Design review of the part built by this model. Coordinates are the model's own, in mm. Face numbers are marked on the shaded views. A direction names the side the tool comes from. Round coordinates to 2 decimals unless told otherwise and drop trailing zeros. Loops run counter-clockwise (first coordinate to the right, second up) from the corner with the lowest first, then second, coordinate; pieces in that order, holes last. Notation, with made-up numbers: M 87.5,40.5 L 134.5,40.5 A21 cw 134.5,73.5 Z; hole C 17.25,10.5 d1. An arc over 180 degrees is marked long. Answer as CSV lines item,"result". Start each with the question number.
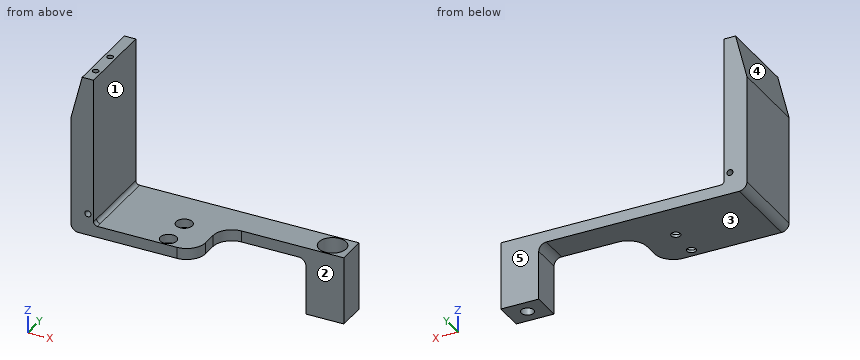
from build123d import *

# Parameters (mm, degrees)
SKETCH_1_W                = 40
SKETCH_1_H                = 10
EXTRUDE_1_DEPTH           = 3
SKETCH_2_W                = 3
SKETCH_2_H                = 10
EXTRUDE_2_DEPTH           = 39.5
EXTRUDE_3_DEPTH           = 10
FILLET_1_R                = 1
SKETCH_4_W                = 40
SKETCH_4_H                = 3
EXTRUDE_4_DEPTH           = 10
HOLE_WIZARD_1_D           = 2.4
HOLE_WIZARD_1_DEPTH       = 3.2
HOLE_WIZARD_1_CBORE_D     = 4.3
HOLE_WIZARD_1_CBORE_DEPTH = 2.3
HOLE_WIZARD_1_TIP         = 0.721032743
HOLE_WIZARD_M2_1_D        = 1.6
HOLE_WIZARD_M2_1_DEPTH    = 5.2
HOLE_WIZARD_M2_1_TIP      = 0.480688495
SKETCH_12_W               = 40
SKETCH_12_H               = 8.5
CUT_EXTRUDE_1_DEPTH       = 43.5
SKETCH_13_W               = 3
SKETCH_13_H               = 21.5
EXTRUDE_5_DEPTH           = 5
SKETCH_14_W               = 3
SKETCH_14_H               = 7.8
EXTRUDE_6_DEPTH           = 27
EXTRUDE_8_DEPTH           = 10
SKETCH_18_W               = 10.684104654
SKETCH_18_H               = 46.640580652
CUT_EXTRUDE_2_DEPTH       = 30
SKETCH_22_W               = 10
SKETCH_22_H               = 7.8
EXTRUDE_9_DEPTH           = 15
SKETCH_23_R               = 3.6
CUT_EXTRUDE_3_DEPTH       = 5
HOLE_WIZARD_M4_1_D        = 3.3
FILLET_2_R                = 2
SKETCH_26_W               = 5
SKETCH_26_H               = 13.7
CUT_EXTRUDE_4_DEPTH       = 8
EXTRUDE_10_DEPTH          = 10
EXTRUDE_11_DEPTH          = 1.5
HOLE_WIZARD_M2_2_D        = 1.6
HOLE_WIZARD_M2_2_DEPTH    = 5.2
HOLE_WIZARD_M2_2_TIP      = 0.480688495
HOLE_WIZARD_M2_3_D        = 1.6
HOLE_WIZARD_M2_3_DEPTH    = 5.2
HOLE_WIZARD_M2_3_TIP      = 0.480688495
HOLE_WIZARD_M2_4_D        = 1.6
HOLE_WIZARD_M2_4_DEPTH    = 5.2
HOLE_WIZARD_M2_4_TIP      = 0.480688495
FILLET_3_R                = 2
FILLET_4_R                = 5


with BuildPart() as part:
    # 草图1 → 凸台-拉伸1 (new body)
    with BuildSketch(Plane.XY):
        Rectangle(SKETCH_1_W, SKETCH_1_H)
    extrude(amount=EXTRUDE_1_DEPTH)

    # 草图2 → 凸台-拉伸2 (add)
    with BuildSketch(Plane.XY.offset(3)):
        with Locations((-8.5, 0)):
            Rectangle(SKETCH_2_W, SKETCH_2_H)
    extrude(amount=EXTRUDE_2_DEPTH)

    # 草图3 → 凸台-拉伸3 (add)
    with BuildSketch(Plane(origin=(0, 5, 0), x_dir=(1, 0, 0), z_dir=(0, 1, 0))):
        Polygon((-20, -3), (-10, -42.5), (-10, -30.276150361), (-16.905354522, -3), align=None)
    extrude(amount=-EXTRUDE_3_DEPTH)

    # 圆角1
    fillet_1_edges = [part.edges().sort_by_distance(p)[0] for p in [
        (-7, 0, 3),
    ]]
    fillet(fillet_1_edges, radius=FILLET_1_R)

    # 草图4 → 凸台-拉伸4 (add)
    with BuildSketch(Plane(origin=(0, 5, 0), x_dir=(1, 0, 0), z_dir=(0, 1, 0))):
        with Locations((0, -1.5)):
            Rectangle(SKETCH_4_W, SKETCH_4_H)
    extrude_4 = extrude(amount=EXTRUDE_4_DEPTH)

    # 镜向1: 凸台-拉伸4 across plane
    add(extrude_4.mirror(Plane.ZX))

    # 打孔尺寸(%根据)内六角圆柱头螺钉的类型1
    with Locations(Plane.XY.offset(3)):
        with Locations((11.5, 4), (11.5, -4)):
            CounterBoreHole(HOLE_WIZARD_1_D / 2, HOLE_WIZARD_1_CBORE_D / 2, HOLE_WIZARD_1_CBORE_DEPTH, depth=HOLE_WIZARD_1_DEPTH)
            with Locations((0, 0, -(HOLE_WIZARD_1_DEPTH + HOLE_WIZARD_1_TIP / 2))):  # 118° drill point
                Cone(0, HOLE_WIZARD_1_D / 2, HOLE_WIZARD_1_TIP, mode=Mode.SUBTRACT)

    # M2 螺纹孔1
    with Locations(Plane.XY.offset(42.5)):
        with Locations((-8.5, -2.5)):
            Hole(HOLE_WIZARD_M2_1_D / 2, depth=HOLE_WIZARD_M2_1_DEPTH)
            with Locations((0, 0, -(HOLE_WIZARD_M2_1_DEPTH + HOLE_WIZARD_M2_1_TIP / 2))):  # 118° drill point
                Cone(0, HOLE_WIZARD_M2_1_D / 2, HOLE_WIZARD_M2_1_TIP, mode=Mode.SUBTRACT)

    # 草图12 → 切除-拉伸1 (cut, through all)
    with BuildSketch(Plane(origin=(0, 0, 0), x_dir=(-1, 0, 0), z_dir=(0, 0, -1))):
        with Locations((0, -10.75)):
            Rectangle(SKETCH_12_W, SKETCH_12_H)
    extrude(amount=-CUT_EXTRUDE_1_DEPTH, mode=Mode.SUBTRACT)

    # 草图13 → 凸台-拉伸5 (add)
    with BuildSketch(Plane(origin=(20, 0, 0), x_dir=(0, 0, -1), z_dir=(1, 0, 0))):
        with Locations((-1.5, 4.25)):
            Rectangle(SKETCH_13_W, SKETCH_13_H)
    extrude(amount=EXTRUDE_5_DEPTH)

    # 草图14 → 凸台-拉伸6 (add)
    with BuildSketch(Plane(origin=(25, 0, 0), x_dir=(0, 0, -1), z_dir=(1, 0, 0))):
        with Locations((-1.5, 11.1)):
            Rectangle(SKETCH_14_W, SKETCH_14_H)
    extrude(amount=EXTRUDE_6_DEPTH)

    # 草图17 → 凸台-拉伸8 (add)
    with BuildSketch(Plane(origin=(0, 5, 0), x_dir=(1, 0, 0), z_dir=(0, 1, 0))):
        Polygon((-16.905354522, -3), (-10, -30.276150361), (-10, -3), align=None)
    extrude(amount=-EXTRUDE_8_DEPTH)

    # 草图18 → 切除-拉伸2 (cut, symmetric)
    with BuildSketch(Plane(origin=(0, 0, 0), x_dir=(1, 0, 0), z_dir=(0, 1, 0))):
        with Locations((-18.342052327, -18.918804504)):
            Rectangle(SKETCH_18_W, SKETCH_18_H)
    extrude(amount=CUT_EXTRUDE_2_DEPTH, both=True, mode=Mode.SUBTRACT)

    # 草图22 → 凸台-拉伸9 (add)
    with BuildSketch(Plane(origin=(0, 0, 0), x_dir=(-1, 0, 0), z_dir=(0, 0, -1))):
        with Locations((-47, 11.1)):
            Rectangle(SKETCH_22_W, SKETCH_22_H)
    extrude(amount=EXTRUDE_9_DEPTH)

    # 草图23 → 切除-拉伸3 (cut)
    with BuildSketch(Plane.XY.offset(3)):
        with Locations((47, 11.1)):
            Circle(SKETCH_23_R)
    extrude(amount=-CUT_EXTRUDE_3_DEPTH, mode=Mode.SUBTRACT)

    # M4 螺纹孔1 (through all)
    with Locations(Plane.XY.offset(-2)):
        with Locations((47, 11.1)):
            Hole(HOLE_WIZARD_M4_1_D / 2)

    # 圆角2
    fillet_2_edges = [part.edges().sort_by_distance(p)[0] for p in [
        (42, 11.1, 0),
    ]]
    fillet(fillet_2_edges, radius=FILLET_2_R)

    # 草图26 → 切除-拉伸4 (cut)
    with BuildSketch(Plane(origin=(0, 0, 0), x_dir=(-1, 0, 0), z_dir=(0, 0, -1))):
        with Locations((-22.5, 0.35)):
            Rectangle(SKETCH_26_W, SKETCH_26_H)
    extrude(amount=-CUT_EXTRUDE_4_DEPTH, mode=Mode.SUBTRACT)

    # 草图27 → 凸台-拉伸10 (add)
    with BuildSketch(Plane(origin=(0, 5, 0), x_dir=(1, 0, 0), z_dir=(0, 1, 0))):
        with BuildLine():
            Line((-6, -3), (-13, -3))
            Line((-13, -3), (-13, -30.65))
            Line((-13, -30.65), (-10, -42.5))
            Line((-10, -42.5), (-7, -42.5))
            Line((-7, -42.5), (-7, -4))
            ThreePointArc((-7, -4), (-6.707106781, -3.292893219), (-6, -3))
        make_face()
    extrude(amount=EXTRUDE_10_DEPTH)

    # 草图28 → 凸台-拉伸11 (add)
    with BuildSketch(Plane.XZ.offset(5)):
        with BuildLine():
            Line((-10, 42.5), (-13, 30.65))
            Line((-13, 30.65), (-13, 3))
            Line((-13, 3), (-6, 3))
            ThreePointArc((-6, 3), (-6.707106781, 3.292893219), (-7, 4))
            Line((-7, 4), (-7, 42.5))
            Line((-7, 42.5), (-10, 42.5))
        make_face()
    extrude(amount=EXTRUDE_11_DEPTH)

    # M2 螺纹孔2
    with Locations(Plane.XY.offset(42.5)):
        with Locations((-8.5, 4.854272417)):
            Hole(HOLE_WIZARD_M2_2_D / 2, depth=HOLE_WIZARD_M2_2_DEPTH)
            with Locations((0, 0, -(HOLE_WIZARD_M2_2_DEPTH + HOLE_WIZARD_M2_2_TIP / 2))):  # 118° drill point
                Cone(0, HOLE_WIZARD_M2_2_D / 2, HOLE_WIZARD_M2_2_TIP, mode=Mode.SUBTRACT)

    # M2 螺纹孔3
    with Locations(Plane(origin=(0, -6.5, 0), x_dir=(-1, 0, 0), z_dir=(0, -1, 0))):
        with Locations((8.5, -5.75)):
            Hole(HOLE_WIZARD_M2_3_D / 2, depth=HOLE_WIZARD_M2_3_DEPTH)
            with Locations((0, 0, -(HOLE_WIZARD_M2_3_DEPTH + HOLE_WIZARD_M2_3_TIP / 2))):  # 118° drill point
                Cone(0, HOLE_WIZARD_M2_3_D / 2, HOLE_WIZARD_M2_3_TIP, mode=Mode.SUBTRACT)

    # M2 螺纹孔4
    with Locations(Plane(origin=(0, 15, 0), x_dir=(1, 0, 0), z_dir=(0, 1, 0))):
        with Locations((-8.5, -5.75)):
            Hole(HOLE_WIZARD_M2_4_D / 2, depth=HOLE_WIZARD_M2_4_DEPTH)
            with Locations((0, 0, -(HOLE_WIZARD_M2_4_DEPTH + HOLE_WIZARD_M2_4_TIP / 2))):  # 118° drill point
                Cone(0, HOLE_WIZARD_M2_4_D / 2, HOLE_WIZARD_M2_4_TIP, mode=Mode.SUBTRACT)

    # 圆角3
    fillet_3_edges = [part.edges().sort_by_distance(p)[0] for p in [
        (-13, 4.25, 0),
    ]]
    fillet(fillet_3_edges, radius=FILLET_3_R)

    # 圆角4
    fillet_4_edges = [part.edges().sort_by_distance(p)[0] for p in [
        (20, 7.2, 1.5),
        (20, -6.5, 1.5),
    ]]
    fillet(fillet_4_edges, radius=FILLET_4_R)


solid = part.part
Item 1: Consider section D-D, the plane z = -9. Write out the cut boundary in (x, y), then the cut area to 3 significant figures.
Item 2: Consider section B-B, the plane x = 11.5. Write out the cut boundary in (y, z).
Item 3: Insertion check: pin 1 Ø6 at (y, z) = (12, 8.5) entering from +X; pin 2 Ø1.4 at (x, y) = (-8.5, 4.85) entering from -Z; pin 3 Ø0.9 at (y, z) = (1, 1.5) entering from +X; pin 4 Ø2 at (x, z) = (10.5, 5.5) entering from +Y. Each pin has a flat end and moves straight along its axis. Give the tip position at first contact, or say it passes through.
Item 4: Consider section A-A, the plane y = 11.1. Write out the cut boundary in (x, z), then the cut area to 3 significant figures.
Item 5: Consider section C-C, the plane x = 47. Write out the cut boundary in (y, z), then the cut area to 3 significant figures.
Item 6: To check wall thickness, follow line 1 (Y direction, x = -8.5, z = 39.15); line 2 (Z direction, x = -5.5, y = 7.25); line 3 (X direction, y = 12, z = 13.5). State the ranges of each line that lie inside material, in increasing order.
Item 7: Tool access review of the marked faces 1, 2, 3, 4 and 5: name each direction out of +Z, -Z, +X, -X, +Y, -Y from which nothing blocks a thin tool from reaching the whole face with its end or side.
Found:
1,outline,"M 42,7.2 L 52,7.2 L 52,15 L 42,15 Z; hole C 47,11.1 d3.3"
1,area,"69.4 mm^2"
2,outline,"M -6.5,0 L -5.2,0 L -5.2,0.7 L -6.15,0.7 L -6.15,3 L -6.5,3 Z; M -2.8,0 L 2.8,0 L 2.8,0.7 L 1.85,0.7 L 1.85,3 L -1.85,3 L -1.85,0.7 L -2.8,0.7 Z; M 5.2,0 L 15,0 L 15,3 L 6.15,3 L 6.15,0.7 L 5.2,0.7 Z"
3,pin 1,"stops at x = -7"
3,pin 2,"stops at z = 0"
3,pin 3,"stops at x = 20"
3,pin 4,"passes through"
4,outline,"M -13,2 A2 ccw -11,0 L 40,0 A2 cw 42,-2 L 42,-15 L 45.35,-15 L 45.35,-2 L 43.4,-2 L 43.4,3 L -6,3 A1 cw -7,4 L -7,42.5 L -10,42.5 L -13,30.65 Z; M 48.65,-15 L 52,-15 L 52,3 L 50.6,3 L 50.6,-2 L 48.65,-2 Z; hole C -8.5,5.75 d1.6"
4,area,"484 mm^2"
5,outline,"M 7.2,-15 L 9.45,-15 L 9.45,-2 L 7.5,-2 L 7.5,3 L 7.2,3 Z; M 12.75,-15 L 15,-15 L 15,3 L 14.7,3 L 14.7,-2 L 12.75,-2 Z"
5,area,"61.5 mm^2"
6,line 1,"y = -6.5 to -3.3, -1.7 to 4.05, 5.65 to 15"
6,line 2,"z = 0 to 3"
6,line 3,"x = -13 to -7"
7,face 1,"+Z, +X, +Y, -Y"
7,face 2,"+Z, -Z, +X, -Y"
7,face 3,"-Z, -X, +Y, -Y"
7,face 4,"+Z, -X, +Y, -Y"
7,face 5,"+Z, -Z, +X, -X, +Y"
